Here's how the part is built. I have some questions about the finished solid (model axes, mm). A direction names the side the tool comes from. Coordinates: 2 decimals unless noted, no trailing zeros. Order: outer loops, then holes, each group sorted by start corner. A loop starts at its lowest first (then second) coordinate and runs counter-clockwise, first axis right, second up. Notation, with made-up numbers: (76, 61) - (85, 61) arc R6 ccw to (85, 65) - close; hole circle Ø6 at (84, 38). An arc over 180 degrees is marked (long way). Answer as CSV lines item,"result". Start each with the question number.
Q1. Suppose I cut it at B-B (x = 0). Count the separate pieces of the cut face and the enclosed holes in it, then the cut area to 3 significant figures.
Q2. Thinking about a two-plate mould opening in Z: for faces 5 (the face through (15.45, 10.87, -4.87)), 6 (the face through (-13, 27, 0)), 7 (the face through (-1.08, 28.77, 4.88)), which applies, released by +Z, released by -Z, zero draft, split by the parting line, or undercut?
Q3. I need wall thicknesses on line 1 (X direction, y = 28, z = 0); line 2 (Y direction, x = -1, z = -10); line 3 (Z direction, x = 0, y = -4.5). Which ranges of each line are inside material? Lowest first, please.
Q4. For faces 1 (the face through (-10.5, 31, 0)), 2 (the face through (14, 27, 0)), 3 (the face through (-9, 35, 0)), 4 (the face through (-9.73, -4.44, 8.92)), which set-ups out of +Z, -Z, +X, -X, +Y, -Y let a thin tool reach every point of the face, with its end or its side?
Q5. For pin 1 Ø3.5 at (y, z) = (33, 0) entering from +X; pin 2 Ø1.7 at (x, z) = (-14, -1.5) entering from +Y; pin 3 Ø6 at (x, y) = (-12.5, -3) entering from -Z, each with a flat end and sliding along its axis, tell me the tip position at first contact or that it passes through.
Q6. Suppose I cut it at A-A (y = 30). Please give me the cut outline in (x, z).
Autodesk Inventor part; units mm, degrees
ref_plane "YZ Plane" through (0, 0, 0) normal (1, 0, 0) x (0, 1, 0)
ref_plane "XZ Plane" through (0, 0, 0) normal (0, 1, 0) x (-1, 0, 0)
ref_plane "XY Plane" through (0, 0, 0) normal (0, 0, 1) x (1, 0, 0)
sketch "Esboço1" plane through (0, 0, 0) normal (0, 0, 1) x (1, 0, 0)
  line L0 (0, 0) -> (14.7, 0)
  line L1 (14.7, 0) -> (16.2, 0)
  line L2 (16.2, 0) -> (16.2, 4.3403)
  line L3 (16.2, 50) -> (14.7, 50)
  line L4 (14.7, 50) -> (13.2, 50)
  line L5 (13.2, 4.3688) -> (13.2, 0)
  line L6 (0, 0) -> (0, 50)
  line L7 (0, 0) -> (5, 0)
  line L8 (5, 28.5381) -> (5, 50)
  line L9 (8, 29) -> (42.1402, 29)
  line L10 (15.5063, 8) -> (35.5749, 8)
  arc A0 (5, 29) -> (11.1701, 10.4085) centre (35.3987, 28.769) ccw
  arc A1 (13.2, 4.3688) -> (11.1701, 10.4085) centre (3.2, 4.3688) ccw
  line L11 (5, 50) -> (8, 50)
  arc A2 (8, 29) -> (14.1456, 10.4122) centre (37.9251, 28.5841) ccw
  arc A3 (16.2, 4.3403) -> (14.1456, 10.4122) centre (6.2, 4.3403) ccw
  line L12 (8, 50) -> (8, 28.1681)
  line L13 (14.7, 0) -> (14.7, 4)
  line L14 (14.7, 9.6081) -> (14.7, 50)
  line L15 (16.2, 4) -> (35.5749, 4)
  line L16 (0, 32) -> (45.564, 32)
  line L17 (16.2, 0) -> (16.2, 50)
  line L18 (8, 29) -> (0, 29)
  line L19 (13.2, 50) -> (13.2, 29)
  line L20 (0, 37) -> (42.1402, 37)
  point P0 (13.2, 8)
  point P1 (16.2, 8)
  point P2 (16.2, 8)
  point P3 (16.2, 29)
  point P4 (8, 32)
  point P5 (5, 32)
  point P6 (5, 29)
  point P7 (16.2, 37)
  point P8 (8, 37)
  point P9 (13.2, 37)
  dimension "d15" = 14.7
  dimension "d16" = 50
  dimension "d17" = 1.5
  dimension "d18" = 1.5
  dimension "d20" = 5
  dimension "d23" = 10
  dimension "d24" = 3
  dimension "d25" = 10
  dimension "d27" = 3
  dimension "d28" = 5
revolve "Revolução1" add sketch "Esboço1" angle 360 about axis through (0, 0, 0) along (0, 1, 0) contours L5 A1 A0 L8 L18 A2 A3 L2 L1 L0 | L9 L14 A3 A2 L12 | L19 L16 L14 L9 | L19 L20 L14 L16 | L14 L16 L17 L9 | L9 L17 L10 A3 L14 | A3 L10 L17 | L14 L20 L17 L16
sketch "Esboço2" plane through (0, 29, 0) normal (0, 1, 0) x (1, 0, 0)
  circle A0 centre (0, 0) radius 13.2
  line L0 (9, -9) -> (-9, -9)
  line L1 (-9, -9) -> (-9, 9)
  line L2 (-9, 9) -> (9, 9)
  line L3 (9, 9) -> (9, -9)
  line L4 (9, -9) -> (-9, 9) construction
  line L5 (-9, -9) -> (9, 9) construction
  dimension "d29" = 18
  dimension "d30" = 18
extrude "Extrusão1" add sketch "Esboço2" along normal blind 8
sketch "Esboço3" plane through (0, 0, 0) normal (0, -1, 0) x (1, 0, 0)
  circle A0 centre (0, 0) radius 13.2
  circle A1 centre (0, 0) radius 16.2
extrude "Extrusão2" add sketch "Esboço3" along normal blind 10
sketch "Esboço4" plane through (0, -10, 0) normal (0, -1, 0) x (1, 0, 0)
  circle A0 centre (0, 0) radius 16.2
  circle A1 centre (0, 0) radius 13.2
extrude "Extrusão3" add sketch "Esboço4" along normal blind 3
sketch "Esboço6" plane through (0, -13, 0) normal (0, -1, 0) x (1, 0, 0)
  circle A0 centre (0, 0) radius 16.2
extrude "Extrusão4" add sketch "Esboço6" along normal blind 3
sketch "Esboço7" plane through (9, 29, -9) normal (-1, 0, 0) x (0, 0, 1)
  circle A0 centre (9, 4) radius 0.5
  line L0 (18, 0) -> (0, 0)
  point P0 (9, -29)
  point P1 (9, 0)
  dimension "d39" = 1
  dimension "d40" = 4
extrude "Extrusão5" cut sketch "Esboço7" against normal blind 43.25
sketch "Esboço9" plane through (0, 37, 0) normal (0, 1, 0) x (1, 0, 0)
  circle A0 centre (0, 0) radius 16.2
  line L0 (-10.5, 12.3365) -> (-10.5, -12.3365)
  line L1 (-9, -9) -> (-9, 9)
  circle A1 centre (0, 0) radius 16.2
  line L2 (12, -10.883) -> (12, 10.883)
  line L3 (9, 9) -> (9, -9)
  dimension "d43" = 1.5
  dimension "d48" = 3
extrude "Extrusão6" cut sketch "Esboço9" against normal blind 10 contours L0 A0
sketch "Esboço10" plane through (9, 29, -9) normal (-1, 0, 0) x (0, 0, 1)
  circle A0 centre (9, 4) radius 0.5
  circle A1 centre (9, 4) radius 1.5
  point P0 (9, -29)
extrude "Extrusão7" cut sketch "Esboço10" along normal blind 43.25 contours A0 | A1
extrude "Extrusão8" cut sketch "Esboço9" against normal blind 10 contours A0 L2
properties part number "Peça2_3DPrint"
Here are the results:
1,separate pieces,"1"
1,enclosed holes,"2"
1,area,"705 mm²"
2,face 5,"split by the parting line"
2,face 6,"zero draft"
2,face 7,"undercut"
3,line 1,"x = -10.5 to -5.01, 5.01 to 12"
3,line 2,"y = -16 to -13, 11.99 to 37"
3,line 3,"z = -16.2 to -13.2, 13.2 to 16.2"
4,face 1,"+Z, -Z, -X, +Y"
4,face 2,"+Z, -Z, +X, +Y"
4,face 3,"+Y"
4,face 4,"none"
5,pin 1,"stops at x = 12"
5,pin 2,"stops at y = 27"
5,pin 3,"stops at z = -13.12"
6,outline,"(-10.5, -12.34) arc R16.2 ccw to (12, -10.88) - (12, 10.88) arc R16.2 ccw to (-10.5, 12.34) - close; hole (-9, -9) - (9, -9) - (9, 9) - (-9, 9) - close"
